The listing builds one solid part. Answer for the finished solid, in the listing's coordinates (mm). Round coordinates to 2 decimals unless told otherwise and drop trailing zeros. Write each loop counter-clockwise with the first axis right and the second up, starting at its lowest first coordinate (ties: lowest second). Pieces come first, ordered by that corner, then holes. Notation, with made-up numbers: (66, 63.5) - (106, 63.5) arc R27 ccw to (106, 81.5) - close; hole circle Ø4 at (84.25, -32.75). An arc over 180 degrees is marked (long way). Answer in a Markdown table with one row per item.
from build123d import *

# Parameters (mm, degrees)
SKETCH2_W                      = 304.8
SKETCH2_H                      = 355.6
MAINBASE_EXTRUDE_DEPTH         = 17.5
SKETCH3_R                      = 15
HOLES_POLE_DEPTH               = 36
M5X0_8_TAPPED_HOLE1_D          = 4.2
M5X0_8_TAPPED_HOLE2_D          = 4.2
M5X0_8_TAPPED_HOLE3_AT_2_COUNT = 2
M5X0_8_TAPPED_HOLE3_AT_2_PITCH = 15
M5X0_8_TAPPED_HOLE3_AT_3_COUNT = 2
M5X0_8_TAPPED_HOLE3_AT_3_PITCH = 57.008771255
M5X0_8_TAPPED_HOLE3_AT_4_COUNT = 2
M5X0_8_TAPPED_HOLE3_AT_4_PITCH = 55
M5X0_8_TAPPED_HOLE3_AT_5_COUNT = 2
M5X0_8_TAPPED_HOLE3_AT_5_PITCH = 115.974135047
M5X0_8_TAPPED_HOLE3_AT_6_COUNT = 2
M5X0_8_TAPPED_HOLE3_AT_6_PITCH = 115
SKETCH14_R                     = 3
CUT_EXTRUDE1_DEPTH             = 10


with BuildPart() as part:
    # Sketch2 → MainBase_Extrude (new body, symmetric)
    with BuildSketch(Plane(origin=(0, 0, 0), x_dir=(1, 0, 0), z_dir=(0, 1, 0))):
        Rectangle(SKETCH2_W, SKETCH2_H)
    extrude(amount=MAINBASE_EXTRUDE_DEPTH, both=True)

    # Sketch3 → Holes_Pole (cut, through all)
    with BuildSketch(Plane(origin=(0, 17.5, 0), x_dir=(1, 0, 0), z_dir=(0, 1, 0))):
        with Locations((-100, 100)):
            Circle(SKETCH3_R)
        with Locations((100, 100)):
            Circle(SKETCH3_R)
        with Locations((100, -100)):
            Circle(SKETCH3_R)
        with Locations((-100, -100)):
            Circle(SKETCH3_R)
    extrude(amount=-HOLES_POLE_DEPTH, mode=Mode.SUBTRACT)

    # M5x0.8 Tapped Hole1 (through all)
    with Locations(Plane(origin=(0, 17.5, 0), x_dir=(1, 0, 0), z_dir=(0, 1, 0))):
        with Locations((-69.85, 19.05), (-19.05, 19.05), (-19.05, -19.05), (-69.85, -19.05), (19.05, 19.05), (19.05, -19.05), (69.85, -19.05), (69.85, 19.05)):
            Hole(M5X0_8_TAPPED_HOLE1_D / 2)

    # M5x0.8 Tapped Hole2 (through all)
    with Locations(Plane(origin=(0, 17.5, 0), x_dir=(1, 0, 0), z_dir=(0, 1, 0))):
        with Locations((-11.5, -45.9918251), (11.5, -45.9918251), (11.5, -85.9918251), (-11.5, -85.9918251), (-11.5, -125.9918251), (11.5, -125.9918251), (-11.5, -165.9918251), (11.5, -165.9918251)):
            m5x0_8_tapped_hole2 = Hole(M5X0_8_TAPPED_HOLE2_D / 2)

    # Mirror1: M5x0.8 Tapped Hole2 across plane
    add(m5x0_8_tapped_hole2.mirror(Plane.XY), mode=Mode.SUBTRACT)

    # Sketch12 → M5x0.8 Tapped Hole3 (revolve, cut)
    with BuildSketch(Plane(origin=(-64.5, -17.5, -142.5), x_dir=(0, 0, -1), z_dir=(1, 0, 0))):
        Polygon((0, 0), (0, 13.6618073), (2.1, 12.4), (2.1, 0), align=None)
    m5x0_8_tapped_hole3 = revolve(axis=Axis((-64.5, -23.85, -142.5), (0, 1, 0)), mode=Mode.SUBTRACT)

    # M5x0.8 Tapped Hole3 at 2: M5x0.8 Tapped Hole3 ×2
    with Locations(*[(i * M5X0_8_TAPPED_HOLE3_AT_2_PITCH, 0, 0) for i in range(1, M5X0_8_TAPPED_HOLE3_AT_2_COUNT)]):
        add(m5x0_8_tapped_hole3, mode=Mode.SUBTRACT)

    # M5x0.8 Tapped Hole3 at 3: M5x0.8 Tapped Hole3 ×2
    with Locations(*[Vector(0.263117406, 0, 0.964763821) * (i * M5X0_8_TAPPED_HOLE3_AT_3_PITCH) for i in range(1, M5X0_8_TAPPED_HOLE3_AT_3_COUNT)]):
        add(m5x0_8_tapped_hole3, mode=Mode.SUBTRACT)

    # M5x0.8 Tapped Hole3 at 4: M5x0.8 Tapped Hole3 ×2
    with Locations(*[(0, 0, i * M5X0_8_TAPPED_HOLE3_AT_4_PITCH) for i in range(1, M5X0_8_TAPPED_HOLE3_AT_4_COUNT)]):
        add(m5x0_8_tapped_hole3, mode=Mode.SUBTRACT)

    # M5x0.8 Tapped Hole3 at 5: M5x0.8 Tapped Hole3 ×2
    with Locations(*[Vector(0.129339184, 0, 0.991600411) * (i * M5X0_8_TAPPED_HOLE3_AT_5_PITCH) for i in range(1, M5X0_8_TAPPED_HOLE3_AT_5_COUNT)]):
        add(m5x0_8_tapped_hole3, mode=Mode.SUBTRACT)

    # M5x0.8 Tapped Hole3 at 6: M5x0.8 Tapped Hole3 ×2
    with Locations(*[(0, 0, i * M5X0_8_TAPPED_HOLE3_AT_6_PITCH) for i in range(1, M5X0_8_TAPPED_HOLE3_AT_6_COUNT)]):
        add(m5x0_8_tapped_hole3, mode=Mode.SUBTRACT)

    # Mirror2: M5x0.8 Tapped Hole3 across plane
    add(m5x0_8_tapped_hole3.mirror(Plane.XY), mode=Mode.SUBTRACT)

    # Mirror2 copy 1 sketch → Mirror2 copy 1 (revolve, cut)
    with BuildSketch(Plane(origin=(-49.5, -17.5, 142.5), x_dir=(0, 0, 1), z_dir=(1, 0, 0))):
        Polygon((0, 0), (0, -13.6618073), (2.1, -12.4), (2.1, 0), align=None)
    revolve(axis=Axis((-49.5, -23.85, 142.5), (0, -1, 0)), mode=Mode.SUBTRACT)

    # Mirror2 copy 2 sketch → Mirror2 copy 2 (revolve, cut)
    with BuildSketch(Plane(origin=(-49.5, -17.5, 87.5), x_dir=(0, 0, 1), z_dir=(1, 0, 0))):
        Polygon((0, 0), (0, -13.6618073), (2.1, -12.4), (2.1, 0), align=None)
    revolve(axis=Axis((-49.5, -23.85, 87.5), (0, -1, 0)), mode=Mode.SUBTRACT)

    # Mirror2 copy 3 sketch → Mirror2 copy 3 (revolve, cut)
    with BuildSketch(Plane(origin=(-64.5, -17.5, 87.5), x_dir=(0, 0, 1), z_dir=(1, 0, 0))):
        Polygon((0, 0), (0, -13.6618073), (2.1, -12.4), (2.1, 0), align=None)
    revolve(axis=Axis((-64.5, -23.85, 87.5), (0, -1, 0)), mode=Mode.SUBTRACT)

    # Mirror2 copy 4 sketch → Mirror2 copy 4 (revolve, cut)
    with BuildSketch(Plane(origin=(-49.5, -17.5, 27.5), x_dir=(0, 0, 1), z_dir=(1, 0, 0))):
        Polygon((0, 0), (0, -13.6618073), (2.1, -12.4), (2.1, 0), align=None)
    revolve(axis=Axis((-49.5, -23.85, 27.5), (0, -1, 0)), mode=Mode.SUBTRACT)

    # Mirror2 copy 5 sketch → Mirror2 copy 5 (revolve, cut)
    with BuildSketch(Plane(origin=(-64.5, -17.5, 27.5), x_dir=(0, 0, 1), z_dir=(1, 0, 0))):
        Polygon((0, 0), (0, -13.6618073), (2.1, -12.4), (2.1, 0), align=None)
    revolve(axis=Axis((-64.5, -23.85, 27.5), (0, -1, 0)), mode=Mode.SUBTRACT)

    # Mirror3: M5x0.8 Tapped Hole3 across plane
    add(m5x0_8_tapped_hole3.mirror(Plane(origin=(0, 0, 0), x_dir=(0, 0, 1), z_dir=(1, 0, 0))), mode=Mode.SUBTRACT)

    # Mirror3 copy 1 sketch → Mirror3 copy 1 (revolve, cut)
    with BuildSketch(Plane(origin=(64.5, -17.5, 142.5), x_dir=(0, 0, 1), z_dir=(-1, 0, 0))):
        Polygon((0, 0), (0, 13.6618073), (2.1, 12.4), (2.1, 0), align=None)
    revolve(axis=Axis((64.5, -23.85, 142.5), (0, 1, 0)), mode=Mode.SUBTRACT)

    # Mirror3 copy 2 sketch → Mirror3 copy 2 (revolve, cut)
    with BuildSketch(Plane(origin=(49.5, -17.5, 142.5), x_dir=(0, 0, 1), z_dir=(-1, 0, 0))):
        Polygon((0, 0), (0, 13.6618073), (2.1, 12.4), (2.1, 0), align=None)
    revolve(axis=Axis((49.5, -23.85, 142.5), (0, 1, 0)), mode=Mode.SUBTRACT)

    # Mirror3 copy 3 sketch → Mirror3 copy 3 (revolve, cut)
    with BuildSketch(Plane(origin=(49.5, -17.5, 87.5), x_dir=(0, 0, 1), z_dir=(-1, 0, 0))):
        Polygon((0, 0), (0, 13.6618073), (2.1, 12.4), (2.1, 0), align=None)
    revolve(axis=Axis((49.5, -23.85, 87.5), (0, 1, 0)), mode=Mode.SUBTRACT)

    # Mirror3 copy 4 sketch → Mirror3 copy 4 (revolve, cut)
    with BuildSketch(Plane(origin=(64.5, -17.5, 87.5), x_dir=(0, 0, 1), z_dir=(-1, 0, 0))):
        Polygon((0, 0), (0, 13.6618073), (2.1, 12.4), (2.1, 0), align=None)
    revolve(axis=Axis((64.5, -23.85, 87.5), (0, 1, 0)), mode=Mode.SUBTRACT)

    # Mirror3 copy 5 sketch → Mirror3 copy 5 (revolve, cut)
    with BuildSketch(Plane(origin=(49.5, -17.5, 27.5), x_dir=(0, 0, 1), z_dir=(-1, 0, 0))):
        Polygon((0, 0), (0, 13.6618073), (2.1, 12.4), (2.1, 0), align=None)
    revolve(axis=Axis((49.5, -23.85, 27.5), (0, 1, 0)), mode=Mode.SUBTRACT)

    # Mirror3 copy 6 sketch → Mirror3 copy 6 (revolve, cut)
    with BuildSketch(Plane(origin=(64.5, -17.5, 27.5), x_dir=(0, 0, 1), z_dir=(-1, 0, 0))):
        Polygon((0, 0), (0, 13.6618073), (2.1, 12.4), (2.1, 0), align=None)
    revolve(axis=Axis((64.5, -23.85, 27.5), (0, 1, 0)), mode=Mode.SUBTRACT)

    # Mirror3 copy 7 sketch → Mirror3 copy 7 (revolve, cut)
    with BuildSketch(Plane(origin=(49.5, -17.5, -142.5), x_dir=(0, 0, -1), z_dir=(-1, 0, 0))):
        Polygon((0, 0), (0, -13.6618073), (2.1, -12.4), (2.1, 0), align=None)
    revolve(axis=Axis((49.5, -23.85, -142.5), (0, -1, 0)), mode=Mode.SUBTRACT)

    # Mirror3 copy 8 sketch → Mirror3 copy 8 (revolve, cut)
    with BuildSketch(Plane(origin=(49.5, -17.5, -87.5), x_dir=(0, 0, -1), z_dir=(-1, 0, 0))):
        Polygon((0, 0), (0, -13.6618073), (2.1, -12.4), (2.1, 0), align=None)
    revolve(axis=Axis((49.5, -23.85, -87.5), (0, -1, 0)), mode=Mode.SUBTRACT)

    # Mirror3 copy 9 sketch → Mirror3 copy 9 (revolve, cut)
    with BuildSketch(Plane(origin=(64.5, -17.5, -87.5), x_dir=(0, 0, -1), z_dir=(-1, 0, 0))):
        Polygon((0, 0), (0, -13.6618073), (2.1, -12.4), (2.1, 0), align=None)
    revolve(axis=Axis((64.5, -23.85, -87.5), (0, -1, 0)), mode=Mode.SUBTRACT)

    # Mirror3 copy 10 sketch → Mirror3 copy 10 (revolve, cut)
    with BuildSketch(Plane(origin=(49.5, -17.5, -27.5), x_dir=(0, 0, -1), z_dir=(-1, 0, 0))):
        Polygon((0, 0), (0, -13.6618073), (2.1, -12.4), (2.1, 0), align=None)
    revolve(axis=Axis((49.5, -23.85, -27.5), (0, -1, 0)), mode=Mode.SUBTRACT)

    # Mirror3 copy 11 sketch → Mirror3 copy 11 (revolve, cut)
    with BuildSketch(Plane(origin=(64.5, -17.5, -27.5), x_dir=(0, 0, -1), z_dir=(-1, 0, 0))):
        Polygon((0, 0), (0, -13.6618073), (2.1, -12.4), (2.1, 0), align=None)
    revolve(axis=Axis((64.5, -23.85, -27.5), (0, -1, 0)), mode=Mode.SUBTRACT)

    # Sketch14 → Cut-Extrude1 (cut)
    with BuildSketch(Plane(origin=(0, 17.5, 0), x_dir=(1, 0, 0), z_dir=(0, 1, 0))):
        with Locations((53.5, 0)):
            Circle(SKETCH14_R)
    cut_extrude1 = extrude(amount=-CUT_EXTRUDE1_DEPTH, mode=Mode.SUBTRACT)

    # Mirror4: Cut-Extrude1 across plane
    add(cut_extrude1.mirror(Plane(origin=(0, 0, 0), x_dir=(0, 0, 1), z_dir=(1, 0, 0))), mode=Mode.SUBTRACT)


solid = part.part
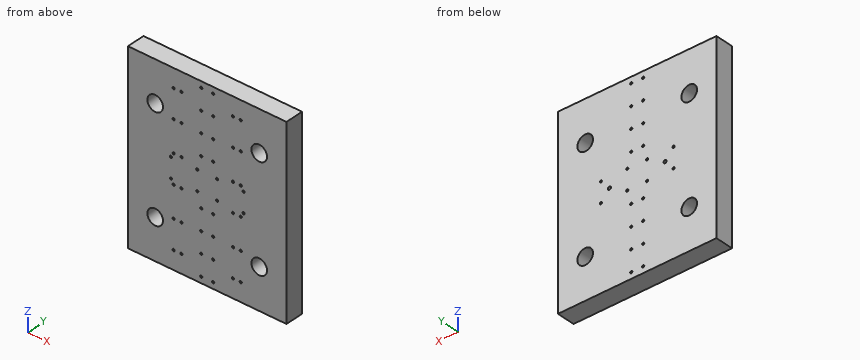
(1) Section B-B (x = 100) is taken. Give the vertices of the cut face in (y, z), and give its area (3 significant figures).
Checked values:
| item | result |
|---|---|
| outline | (-17.5, -177.8) - (17.5, -177.8) - (17.5, -115) - (-17.5, -115) - close; (-17.5, -85) - (17.5, -85) - (17.5, 85) - (-17.5, 85) - close; (-17.5, 115) - (17.5, 115) - (17.5, 177.8) - (-17.5, 177.8) - close |
| area | 10,300 mm2 |
(2) Flat-ended cylindrical pins translate along their axes: pin 1 (1.8 mm diameter, centred on x = -53.5, z = 1, fed in from +Y); pin 2 (4 mm diameter, centred on x = 64.5, z = -142.5, fed in from -Y); pin 3 (4 mm diameter, centred on x = -11.5, z = -45.99, fed in from +Y). Find the tip coordinate at first contact, or state that the pin passes through.
Checked values:
| item | result |
|---|---|
| pin 1 | stops at y = 7.5 |
| pin 2 | stops at y = -5.04 |
| pin 3 | passes through |
(3) Section C-C (y = 3) is taken. State how many separate pieces and enclosed holes the cut face has, and give its area (3 significant figures).
Checked values:
| item | result |
|---|---|
| separate pieces | 1 |
| enclosed holes | 28 |
| area | 105,000 mm2 |
(4) Section A-A (z = -100) is taken. Give the vertices of the cut face in (x, y), and give its area (3 significant figures).
Checked values:
| item | result |
|---|---|
| outline | (-152.4, -17.5) - (-115, -17.5) - (-115, 17.5) - (-152.4, 17.5) - close; (-85, -17.5) - (85, -17.5) - (85, 17.5) - (-85, 17.5) - close; (115, -17.5) - (152.4, -17.5) - (152.4, 17.5) - (115, 17.5) - close |
| area | 8,570 mm2 |
(5) Find the intervals of material crossed by line 1 (X direction, y = -10, z = -142); line 2 (X direction, y = -7, z = 100.5); line 3 (Z direction, x = -69.5, y = 11.5), in increasing order.
Checked values:
| item | result |
|---|---|
| line 1 | x = -152.4 to -66.54, -62.46 to -51.54, -47.46 to 47.46, 51.54 to 62.46, 66.54 to 152.4 |
| line 2 | x = -152.4 to -114.99, -85.01 to 85.01, 114.99 to 152.4 |
| line 3 | z = -177.8 to -21.12, -16.98 to 16.98, 21.12 to 177.8 |
